CAD build for the part. Positions are in the model's coordinates, mm. Face numbers are marked on the shaded views. A direction names the side the tool comes from. Round coordinates to 2 decimals unless told otherwise and drop trailing zeros. Write each loop counter-clockwise with the first axis right and the second up, starting at its lowest first coordinate (ties: lowest second). Pieces come first, ordered by that corner, then holes. Notation, with made-up numbers: (49.5, 35.5) - (90.5, 35.5) arc R35 cw to (90.5, 74.5) - close; hole circle Ø10 at (-10, -32). An arc over 180 degrees is marked (long way). Use one line per item in the form item = value. Start each with the question number.
Item 1: Band-saw the part on A-A, the plane z = 11. List the corners of the cut face in (x, y), and give its area (3 significant figures).
Item 2: Band-saw the part on B-B, the plane y = -119. List the corners of the cut face in (x, z).
Item 3: Pin check, flat tips, straight feed: pin 1 (1.7 mm diameter, centred on x = 0, y = 0, fed in from -Z); pin 2 (5 mm diameter, centred on x = 2.5, z = 12.5, fed in from -Y); pin 3 (12 mm diameter, centred on x = -3, z = 19, fed in from +Y); pin 4 (4 mm diameter, centred on x = -1, y = -0.5, fed in from +Z). Stop position of each tip, or through.
Item 4: Band-saw the part on C-C, the plane x = 0. Give the number of separate pieces and of enclosed holes in the cut face, and give its area (3 significant figures).
Item 5: Pull direction Z, two halves, no side cores. Call the marked faces 1, 2 and 3: +Z half, -Z half, draft (parallel to the pull), parting line (faces both ways), or undercut.
Item 6: Band-saw the part on D-D, the plane y = -39. List the corners of the cut face in (x, z), and give its area (3 significant figures).
Item 7: Tool access for the marked faces 4 and 5: list every direction of +Z, -Z, +X, -X, +Y, -Y with a clear straight run to the whole face (end or side of a thin tool).
Item 8: Drill centre lines: L1, parallel to Y at x = 0, z = 5.9; L2, parallel to Y at x = 0, z = 11.5; L3, parallel to Y at x = 0, z = 23.35. Where is each one in solid material? Low to high.
from build123d import *

# Parameters (mm, degrees)
SKETCH_1_R               = 10
EXTRUDE_1_DEPTH          = 28
EXTRUDE_START            = -15
EXTRUDE_2_DEPTH          = 15
CUT_EXTRUDE_2_DEPTH      = 128.720701533
CUT_EXTRUDE_2_DEPTH_BACK = 128.720701533
SKETCH_3_R               = 4
CUT_EXTRUDE_3_DEPTH      = 129.412129246
CUT_EXTRUDE_3_DEPTH_BACK = 129.412129246
SKETCH_7_W               = 10
SKETCH_7_H               = 22
CUT_EXTRUDE_4_DEPTH      = 128.428989534
CUT_EXTRUDE_4_DEPTH_BACK = 128.428989534
SKETCH_8_R               = 3
EXTRUDE_START_2          = -3
SKETCH_9_R               = 4
EXTRUDE_3_DEPTH          = 3
SKETCH_10_R              = 1.4
CUT_EXTRUDE_5_DEPTH      = 128.267326381
CHAMFER_1_SIZE           = 0.5


with BuildPart() as part:
    # 草图1 → 凸台-拉伸1 (new body)
    with BuildSketch(Plane.XY):
        Circle(SKETCH_1_R)
    extrude(amount=EXTRUDE_1_DEPTH)

    # 草图2 → 凸台-拉伸2 (add)
    with BuildSketch(Plane.XY.offset(20).offset(EXTRUDE_START)):
        with BuildLine():
            Line((-9.998718605, -0.160082009), (-8, -125))
            Line((-8, -125), (8, -125))
            Line((8, -125), (9.842868133, -1.765770913))
            ThreePointArc((9.842868133, -1.765770913), (-0.806617354, -9.967415334), (-9.998718605, -0.160082009))
        make_face()
    extrude(amount=EXTRUDE_2_DEPTH)

    # 草图3 → 切除-拉伸2 (cut, two sides: drawn at the far end of the back side and taken through both)
    with BuildSketch(Plane(origin=(0, 0, 3.76), x_dir=(-1, 0, 0), z_dir=(0, 0, -1)).offset(-CUT_EXTRUDE_2_DEPTH_BACK)):
        Circle(SKETCH_3_R)
    extrude(amount=CUT_EXTRUDE_2_DEPTH + CUT_EXTRUDE_2_DEPTH_BACK, mode=Mode.SUBTRACT)

    # 切除-放样2: read off the stored shape, not the designer's step
    # 切除-放样2: loft between two sections, ruled curve by curve
    loft_2_from = [
        Edge.make_bspline([(3.291276386, -2.27321353, 3.76), (-1.255150675, -8.855766301, 3.76), (-7.837703446, -4.309339241, 3.76), (-3.291276386, 2.27321353, 3.76), (1.255150675, 8.855766301, 3.76), (7.837703446, 4.309339241, 3.76), (3.291276386, -2.27321353, 3.76)], [0, 0, 0, 0, 0.5, 0.5, 0.5, 1, 1, 1, 1], 3, [1, 0.333333333, 0.333333333, 1, 0.333333333, 0.333333333, 1]),
    ]
    loft_2_to = [
        Edge.make_bspline([(6.471228023, 8.895122702, 0), (24.261473426, -4.047333344, 0), (11.319017381, -21.837578747, 0), (-6.471228023, -8.895122702, 0), (-24.261473426, 4.047333344, 0), (-11.319017381, 21.837578747, 0), (6.471228023, 8.895122702, 0)], [0, 0, 0, 0, 0.5, 0.5, 0.5, 1, 1, 1, 1], 3, [1, 0.333333333, 0.333333333, 1, 0.333333333, 0.333333333, 1]),
    ]
    loft_2 = Solid(Shell([*[Face.make_surface_from_curves(loft_2_from[k], loft_2_to[k]) for k in range(1)], Face(Wire(loft_2_from)), Face(Wire(loft_2_to))]))
    add(loft_2, mode=Mode.SUBTRACT)

    # 镜向1: 切除-放样2 across plane
    add(loft_2.mirror(Plane(origin=(0, 0, 14), x_dir=(1, 0, 0), z_dir=(0, 0, -1))), mode=Mode.SUBTRACT)

    # 草图7 → 切除-拉伸3 (cut, two sides: drawn at the far end of the back side and taken through both)
    with BuildSketch(Plane(origin=(0, 0, 0), x_dir=(0, 0, -1), z_dir=(1, 0, 0)).offset(-CUT_EXTRUDE_3_DEPTH_BACK)):
        with Locations((-12.5, -119)):
            Rectangle(SKETCH_7_W, SKETCH_7_H)
    extrude(amount=CUT_EXTRUDE_3_DEPTH + CUT_EXTRUDE_3_DEPTH_BACK, mode=Mode.SUBTRACT)

    # 草图8 → 切除-拉伸4 (cut, two sides: drawn at the far end of the back side and taken through both)
    with BuildSketch(Plane(origin=(0, 0, 5), x_dir=(-1, 0, 0), z_dir=(0, 0, -1)).offset(-CUT_EXTRUDE_4_DEPTH_BACK)):
        with Locations((0, -119)):
            Circle(SKETCH_8_R)
    extrude(amount=CUT_EXTRUDE_4_DEPTH + CUT_EXTRUDE_4_DEPTH_BACK, mode=Mode.SUBTRACT)

    # 草图9 → 凸台-拉伸3 (add)
    with BuildSketch(Plane.XY.offset(25.072168523).offset(EXTRUDE_START_2)):
        with Locations(Location((0, 0, 0), (0, 0, 180))):
            Circle(SKETCH_9_R)
    extrude(amount=EXTRUDE_3_DEPTH)

    # 草图10 → 切除-拉伸5 (cut, through all)
    with BuildSketch(Plane(origin=(0, 0, 22.072168523), x_dir=(-1, 0, 0), z_dir=(0, 0, -1))):
        Circle(SKETCH_10_R)
    extrude(amount=-CUT_EXTRUDE_5_DEPTH, mode=Mode.SUBTRACT)

    # 倒角1
    chamfer_1_edges = [part.edges().sort_by_distance(p)[0] for p in [
        (3, -119, 7.5),
        (3, -119, 5),
        (3, -119, 20),
        (3, -119, 17.5),
    ]]
    chamfer(chamfer_1_edges, length=CHAMFER_1_SIZE)


solid = part.part
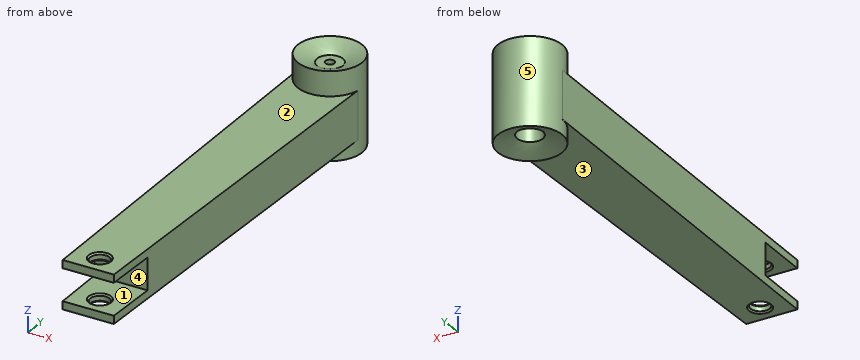
Determined:
q1.outline = (-10, -0.16) - (-8.27, -108) - (8.25, -108) - (9.84, -1.77) arc R10 ccw (long way) to start; hole circle Ø8 at (0, 0)
q1.area = 2,070 mm²
q2.outline = (-8.1, 5) - (-3.5, 5) - (-3, 5.5) - (-3, 7) - (-3.5, 7.5) - (-8.1, 7.5) - close; (-8.1, 17.5) - (-3.5, 17.5) - (-3, 18) - (-3, 19.5) - (-3.5, 20) - (-8.1, 20) - close; (3, 5.5) - (3.5, 5) - (8.09, 5) - (8.09, 7.5) - (3.5, 7.5) - (3, 7) - close; (3, 18) - (3.5, 17.5) - (8.09, 17.5) - (8.09, 20) - (3.5, 20) - (3, 19.5) - close
q3.pin_1 = through
q3.pin_2 = -108
q3.pin_3 = 10
q3.pin_4 = 25.07
q4.separate_pieces = 4
q4.enclosed_holes = 0
q4.area = 1,840 mm²
q5.face_1 = undercut
q5.face_2 = +Z half
q5.face_3 = -Z half
q6.outline = (-9.38, 5) - (9.29, 5) - (9.29, 20) - (-9.38, 20) - close
q6.area = 280 mm²
q7.face_4 = +X, -X, -Y
q7.face_5 = none
q8.L1 = -125 to -122, -116 to -4, 4 to 10
q8.L2 = -108 to -4, 4 to 10
q8.L3 = -10 to -1.4, 1.4 to 10
